from build123d import *

# Parameters (mm, degrees)
F0_R     = 13.45
F1_DEPTH = 63
F2_R     = 9.5
F3_DEPTH = 63.001
F4_R     = 10.3
F5_DEPTH = 10


with BuildPart() as f1:
    # F0 (on Right) → F1 (new body)
    with BuildSketch(Plane.YZ):
        Circle(F0_R)
    extrude(amount=F1_DEPTH)

    # F2 (on face) → F3 (cut, through all)
    with BuildSketch(Plane.YZ.offset(63)):
        Circle(F2_R)
    extrude(amount=-F3_DEPTH, mode=Mode.SUBTRACT)

    # F4 (on face) → F5 (cut)
    with BuildSketch(Plane.YZ.offset(63)):
        Circle(F4_R)
    extrude(amount=-F5_DEPTH, mode=Mode.SUBTRACT)


solid = f1.part
Geometry: final body of the model. Coordinates: model frame, mm. A direction names the side the tool comes from. Round coordinates to 2 decimals unless told otherwise and drop trailing zeros. Order: outer loops, then holes, each group sorted by start corner. A loop starts at its lowest first (then second) coordinate and runs counter-clockwise, first axis right, second up. Notation, with made-up numbers: (-9, -27) - (28, -27) arc R20 ccw to (28, -2) - close; hole circle Ø6 at (-3, 30). An arc over 180 degrees is marked (long way). Write each question's results on one line, items separated by ' | '.
Item 1: Section D-D, the plane x = 56.5. Return the cut outline in (y, z).
Completed:
outline: circle Ø26.9 at (0, 0); hole circle Ø20.6 at (0, 0)
Item 2: Section C-C, the plane x = 18.5. Return the cut outline in (y, z), and give its area (3 significant figures).
Completed:
outline: circle Ø26.9 at (0, 0); hole circle Ø19 at (0, 0) | area: 285 mm^2
Item 3: Reachability of faces 1 (the flat face through (53, 7, -7)), 2 (the flat face through (63, 7, -8)) from +Z, -Z, +X, -X, +Y, -Y: full face, straight path, thin tool, end or side. Return the list, or none.
Completed:
face 1: +X | face 2: +Z, -Z, +X, +Y, -Y
Item 4: Mould query, pull axis Z, two halves, no side actions, for faces 3 (the flat face through (0, -3.2, 9.2)), 4 (the cylindrical face through (58.07, 9.824, 3.094)), 5 (the cylindrical face through (31.06, 12.83, 4.04)). Classes: pulls with the +Z half, pulls with the -Z half, needs draft (parallel to the pull), parting line crosses it, or undercut.
Completed:
face 3: needs draft | face 4: undercut | face 5: parting line crosses it
Item 5: Material intervals for line 1 along Z through (x, y) = (17.5, -0.5); line 2 along Z through (x, y) = (58.5, 0); line 3 along Y through (x, z) = (24, -2), sorted ascending. Write a range as [from, to].
Completed:
line 1: [-13.44, -9.49], [9.49, 13.44] | line 2: [-13.45, -10.3], [10.3, 13.45] | line 3: [-13.3, -9.29], [9.29, 13.3]
Item 6: First-contact query: pin 1 Ø10 at (x, z) = (56, -6.5) entering from -Y; pin 2 Ø1 at (x, y) = (13.5, 9) entering from -Z; pin 3 Ø12 at (x, z) = (33, -7) entering from +Y; pin 4 Ø4 at (y, z) = (-4.5, -8.5) entering from -X. Flat tips, straight axial feed; report the tip coordinate or a pass-through.
Completed:
pin 1: y = -13.37 | pin 2: z = -10.42 | pin 3: y = 13.41 | pin 4: x = 0
Item 7: Section A-A, the plane y = 0. Return the cut outline in (x, z), and give its area (3 significant figures).
Completed:
outline: (0, -13.45) - (63, -13.45) - (63, -10.3) - (53, -10.3) - (53, -9.5) - (0, -9.5) - close; (0, 9.5) - (53, 9.5) - (53, 10.3) - (63, 10.3) - (63, 13.45) - (0, 13.45) - close | area: 482 mm^2
